Can you work these out from the model? Positions are in its coordinate system, mm. Give positions to 0.01 mm unless a question says otherwise; leave off trailing zeros. Write each loop counter-clockwise with the first axis right and the second up, starting at its lowest first coordinate (ties: lowest second). Pieces come first, ordered by that corner, then holes. Notation, with made-up numbers: (51, 45.5) -> (56, 45.5) arc R36 cw to (56, 80.5) -> close; hole circle Ø5 at (33.5, 5). An arc over 180 degrees is marked (long way). Answer as CSV lines item,"result". Start each with the question number.
1. I'm going to push flat-ended pins straight in: P1, Ø1.5, axis at y = 16, z = 1.5, coming from the +X side; P2, Ø2.5, axis at x = 108, z = 2.5, coming from the +Y side; P3, Ø2.5, axis at y = 17, z = 1.5, coming from the -X side. Where does each tip first touch, or does it pass through?
2. If we section it at A-A on x = 22.5: Write out the boundary of the cut face in (y, z) (3 decimals), plus the area to 4 significant figures.
3. If we section it at C-C on z = 1.35: Write out the boundary of the cut face in (x, y) (3 decimals), plus the area to 3 significant figures.
4. If we section it at D-D on x = -22.5: Write out the boundary of the cut face in (y, z) (3 decimals), plus the area to 3 significant figures.
5. I need wall thicknesses on line 1 (Y direction, x = 95, z = 1.9); line 2 (Y direction, x = 22.5, z = 2.05) (3 decimals); line 3 (Y direction, x = -22.5, z = 3.95) (3 decimals). Which ranges of each line are inside material? Lowest first, please. Write a range as [from, to].
6. If we section it at B-B on y = -25: Write out the boundary of the cut face in (x, z) (3 decimals), plus the area to 3 significant figures.
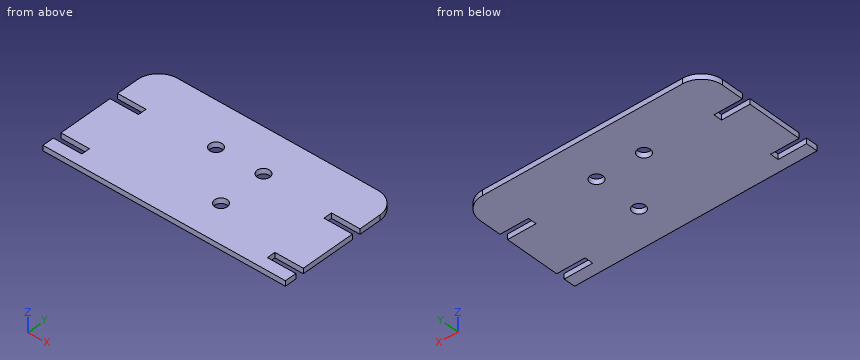
```python
from build123d import *

# Parameters (mm, degrees)
SKETCH1_W           = 230
SKETCH1_H           = 120
BOSS_EXTRUDE1_DEPTH = 5
CUT_EXTRUDE1_REACH  = 131.808
SKETCH2_W           = 27
SKETCH2_H           = 8.000000001
CUT_EXTRUDE2_REACH  = 131.808
SKETCH3_R           = 6.025
FILLET1_R           = 20


with BuildPart() as part:
    # Sketch1 → Boss-Extrude1 (new body)
    with BuildSketch(Plane.XY):
        Rectangle(SKETCH1_W, SKETCH1_H)
    extrude(amount=BOSS_EXTRUDE1_DEPTH)

    # Sketch2 → Cut-Extrude1 (cut, up to next)
    with BuildSketch(Plane(origin=(0, 0, 0), x_dir=(-1, 0, 0), z_dir=(0, 0, -1)), mode=Mode.PRIVATE) as cut_extrude1_sk1:
        with Locations((101.5, 15.000000001)):
            Rectangle(SKETCH2_W, SKETCH2_H)
    cut_extrude1_tool1 = extrude(cut_extrude1_sk1.sketch, amount=-CUT_EXTRUDE1_REACH, mode=Mode.PRIVATE) & part.part
    # Sketch2 → Cut-Extrude1 (cut, up to next)
    with BuildSketch(Plane(origin=(0, 0, 0), x_dir=(-1, 0, 0), z_dir=(0, 0, -1)), mode=Mode.PRIVATE) as cut_extrude1_sk2:
        with Locations((101.5, -45.000000001)):
            Rectangle(SKETCH2_W, SKETCH2_H)
    cut_extrude1_tool2 = extrude(cut_extrude1_sk2.sketch, amount=-CUT_EXTRUDE1_REACH, mode=Mode.PRIVATE) & part.part
    # Sketch2 → Cut-Extrude1 (cut, up to next)
    with BuildSketch(Plane(origin=(0, 0, 0), x_dir=(-1, 0, 0), z_dir=(0, 0, -1)), mode=Mode.PRIVATE) as cut_extrude1_sk3:
        with Locations((-101.5, -45.000000001)):
            Rectangle(SKETCH2_W, SKETCH2_H)
    cut_extrude1_tool3 = extrude(cut_extrude1_sk3.sketch, amount=-CUT_EXTRUDE1_REACH, mode=Mode.PRIVATE) & part.part
    # Sketch2 → Cut-Extrude1 (cut, up to next)
    with BuildSketch(Plane(origin=(0, 0, 0), x_dir=(-1, 0, 0), z_dir=(0, 0, -1)), mode=Mode.PRIVATE) as cut_extrude1_sk4:
        with Locations((-101.5, 15.000000001)):
            Rectangle(SKETCH2_W, SKETCH2_H)
    cut_extrude1_tool4 = extrude(cut_extrude1_sk4.sketch, amount=-CUT_EXTRUDE1_REACH, mode=Mode.PRIVATE) & part.part
    add(cut_extrude1_tool1.solids().sort_by_distance((-101.5, 15, 0))[0], mode=Mode.SUBTRACT)
    add(cut_extrude1_tool2.solids().sort_by_distance((-101.5, -45, 0))[0], mode=Mode.SUBTRACT)
    add(cut_extrude1_tool3.solids().sort_by_distance((101.5, -45, 0))[0], mode=Mode.SUBTRACT)
    add(cut_extrude1_tool4.solids().sort_by_distance((101.5, 15, 0))[0], mode=Mode.SUBTRACT)

    # Sketch3 → Cut-Extrude2 (cut, up to next)
    with BuildSketch(Plane.XY.offset(5), mode=Mode.PRIVATE) as cut_extrude2_sk1:
        with Locations((22.5, 20)):
            Circle(SKETCH3_R)
    cut_extrude2_tool1 = extrude(cut_extrude2_sk1.sketch, amount=-CUT_EXTRUDE2_REACH, mode=Mode.PRIVATE) & part.part
    # Sketch3 → Cut-Extrude2 (cut, up to next)
    with BuildSketch(Plane.XY.offset(5), mode=Mode.PRIVATE) as cut_extrude2_sk2:
        with Locations((-22.5, 20)):
            Circle(SKETCH3_R)
    cut_extrude2_tool2 = extrude(cut_extrude2_sk2.sketch, amount=-CUT_EXTRUDE2_REACH, mode=Mode.PRIVATE) & part.part
    # Sketch3 → Cut-Extrude2 (cut, up to next)
    with BuildSketch(Plane.XY.offset(5), mode=Mode.PRIVATE) as cut_extrude2_sk3:
        with Locations((22.5, -25)):
            Circle(SKETCH3_R)
    cut_extrude2_tool3 = extrude(cut_extrude2_sk3.sketch, amount=-CUT_EXTRUDE2_REACH, mode=Mode.PRIVATE) & part.part
    add(cut_extrude2_tool1.solids().sort_by_distance((22.5, 20, 5))[0], mode=Mode.SUBTRACT)
    add(cut_extrude2_tool2.solids().sort_by_distance((-22.5, 20, 5))[0], mode=Mode.SUBTRACT)
    add(cut_extrude2_tool3.solids().sort_by_distance((22.5, -25, 5))[0], mode=Mode.SUBTRACT)

    # Fillet1
    fillet1_edges = [part.edges().sort_by_distance(p)[0] for p in [
        (-115, 60, 2.5),
        (115, 60, 2.5),
    ]]
    fillet(fillet1_edges, radius=FILLET1_R)


solid = part.part
```
Computed values:
1,P1,"stops at x = 88"
1,P2,"stops at y = 56.18"
1,P3,"stops at x = -88"
2,outline,"(-60, 0) -> (-31.025, 0) -> (-31.025, 5) -> (-60, 5) -> close; (-18.975, 0) -> (13.975, 0) -> (13.975, 5) -> (-18.975, 5) -> close; (26.025, 0) -> (60, 0) -> (60, 5) -> (26.025, 5) -> close"
2,area,"479.5 mm2"
3,outline,"(-115, -60) -> (115, -60) -> (115, -49) -> (88, -49) -> (88, -41) -> (115, -41) -> (115, 11) -> (88, 11) -> (88, 19) -> (115, 19) -> (115, 40) arc R20 ccw to (95, 60) -> (-95, 60) arc R20 ccw to (-115, 40) -> (-115, 19) -> (-88, 19) -> (-88, 11) -> (-115, 11) -> (-115, -41) -> (-88, -41) -> (-88, -49) -> (-115, -49) -> close; hole circle Ø12.05 at (-22.5, 20); hole circle Ø12.05 at (22.5, -25); hole circle Ø12.05 at (22.5, 20)"
3,area,"26,200 mm2"
4,outline,"(-60, 0) -> (13.975, 0) -> (13.975, 5) -> (-60, 5) -> close; (26.025, 0) -> (60, 0) -> (60, 5) -> (26.025, 5) -> close"
4,area,"540 mm2"
5,line 1,"y = [-60, -49], [-41, 11], [19, 60]"
5,line 2,"y = [-60, -31.025], [-18.975, 13.975], [26.025, 60]"
5,line 3,"y = [-60, 13.975], [26.025, 60]"
6,outline,"(-115, 0) -> (16.475, 0) -> (16.475, 5) -> (-115, 5) -> close; (28.525, 0) -> (115, 0) -> (115, 5) -> (28.525, 5) -> close"
6,area,"1,090 mm2"
